from build123d import *

# Parameters (mm, degrees)
SKETCH2_W = 2.3876
SKETCH2_H = 7.239


with BuildPart() as part:
    # Sweep1: sweep along a path in Sketch1
    with BuildLine(Plane.XY) as sweep1_path:
        Line((-97.917, 85.217), (97.917, 85.217))
        Line((97.917, 85.217), (97.917, -85.217))
        Line((97.917, -85.217), (-97.917, -85.217))
        Line((-97.917, -85.217), (-97.917, 85.217))
    # Sketch2 → Sweep1 (sweep)
    with BuildSketch(Plane(origin=(0, 0, 0), x_dir=(0, 0, -1), z_dir=(1, 0, 0))):
        with Locations((-1.1938, 85.217)):
            Rectangle(SKETCH2_W, SKETCH2_H)
    sweep(path=sweep1_path.line, transition=Transition.RIGHT)


solid = part.part
Build history of the part. All positions in model axes, mm. Round coordinates to 2 decimals unless told otherwise and drop trailing zeros. Write each loop counter-clockwise with the first axis right and the second up, starting at its lowest first coordinate (ties: lowest second). Pieces come first, ordered by that corner, then holes. Notation, with made-up numbers: M 21,60 L 39,60 A15 cw 39,74 Z; hole C -29.5,51 d4. An arc over 180 degrees is marked long. Answer as a JSON object with one key per item and string values. Group by question number.
(1) Cut at B-B (y = 37). Give the cut face in (x, z).
(2) Cut at A-A (z = 1.85). Give the cut face in (x, y).
(3) Drill centre lines: L1, parallel to X at y = 48.5, z = 1.35; L2, parallel to Y at x = -73, z = 0.45. Where is each one in solid material? Low to high.
(4) Cut at C-C (x = 82.5). Give the cut face in (y, z), and give its area (3 significant figures).
Responses:
{
 "1": {"outline": "M -101.54,0 L -94.3,0 L -94.3,2.39 L -101.54,2.39 Z; M 94.3,0 L 101.54,0 L 101.54,2.39 L 94.3,2.39 Z"},
 "2": {"outline": "M -101.54,-88.84 L 101.54,-88.84 L 101.54,88.84 L -101.54,88.84 Z; hole M -94.3,-81.6 L 94.3,-81.6 L 94.3,81.6 L -94.3,81.6 Z"},
 "3": {"L1": "x = -101.54 to -94.3, 94.3 to 101.54", "L2": "y = -88.84 to -81.6, 81.6 to 88.84"},
 "4": {"outline": "M -88.84,0 L -81.6,0 L -81.6,2.39 L -88.84,2.39 Z; M 81.6,0 L 88.84,0 L 88.84,2.39 L 81.6,2.39 Z", "area": "34.6 mm2"}
}
